Build history of the part. All positions in model axes, mm. A direction names the side the tool comes from. Give positions to 0.01 mm unless a question says otherwise; leave off trailing zeros. Write each loop counter-clockwise with the first axis right and the second up, starting at its lowest first coordinate (ties: lowest second). Pieces come first, ordered by that corner, then holes. Notation, with made-up numbers: (1.25, -1.5) -> (8.25, -1.5) arc R18 ccw to (8.25, 11.5) -> close; hole circle Ø4 at (81.5, 77). An arc over 180 degrees is marked (long way). Put each result on its own line as item: value. Start each with the question number.
Item 1: Slice it at A-A, the plane z = 28.5. List the corners of the cut face in (x, y).
Item 2: Two-plate mould, pull along X, no slides. Class faces 1 (the flat face through (-90.694, 2, 25)), 2 (the flat face through (-110, 2, 20.456)), 3 (the flat face through (-103, 3, 21.956)): pulls with the +X half, pulls with the -X half, needs draft (parallel to the pull), parting line crosses it, or undercut.
Item 3: Slice it at C-C, the plane z = 23.5. List the corners of the cut face in (x, y), plus the area to 3 significant figures.
Item 4: Slice it at B-B, the plane x = -95.25. List the corners of the cut face in (y, z).
Item 5: Flat gauge pins, fed straight in: pin 1 Ø4.5 at (x, z) = (-95.19, 24.96) entering from +Y; pin 2 Ø1.5 at (x, y) = (-103.5, 3) entering from -Z. Where does each tip first touch, or does it go through?
Item 6: Tool access for faces 4 (the flat face through (-99.694, 3, 21)), 5 (the flat face through (-95, 2, 29.456)), 6 (the flat face through (-99.694, 3, 29)): list every direction of +Z, -Z, +X, -X, +Y, -Y with a clear straight run to the whole face (end or side of a thin tool).
Item 7: Slice it at D-D, the plane y = 2.05. List the corners of the cut face in (x, z), plus the area to 3 significant figures.
Item 8: Drill centre lines: line 1 along X through (y, z) = (3.2, 26); line 2 along X through (y, z) = (1.55, 21.75); line 3 along X through (y, z) = (0.7, 24.75). Where is each one in solid material? Low to high.
```python
from build123d import *

# Parameters (mm, degrees)
SKETCH3_W           = 24
SKETCH3_H           = 9
BOSS_EXTRUDE2_DEPTH = 5
SKETCH4_R           = 1.7
SKETCH4_R_2         = 1
SKETCH4_W           = 6
SKETCH4_H           = 1.5
CUT_EXTRUDE1_DEPTH  = 5


with BuildPart() as part:
    # Sketch3 → Boss-Extrude2 (new body)
    with BuildSketch(Plane(origin=(0, 0, 0), x_dir=(1, 0, 0), z_dir=(0, 1, 0))):
        with Locations((-102.694405771, -24.955608755)):
            Rectangle(SKETCH3_W, SKETCH3_H)
    extrude(amount=BOSS_EXTRUDE2_DEPTH)

    # Sketch4 → Cut-Extrude1 (cut)
    with BuildSketch(Plane(origin=(0, 5, 0), x_dir=(1, 0, 0), z_dir=(0, 1, 0))):
        with Locations((-110.194405771, -24.955608755)):
            Circle(SKETCH4_R)
        with Locations((-95.194405771, -24.955608755)):
            Circle(SKETCH4_R)
        with Locations((-102.694405771, -24.955608755)):
            Circle(SKETCH4_R_2)
        with Locations((-102.694405771, -28.705608755)):
            Rectangle(SKETCH4_W, SKETCH4_H)
        with Locations((-102.694405771, -21.205608755)):
            Rectangle(SKETCH4_W, SKETCH4_H)
    extrude(amount=-CUT_EXTRUDE1_DEPTH, mode=Mode.SUBTRACT)


solid = part.part
```
Values follow:
1. outline: (-114.69, 0) -> (-105.69, 0) -> (-105.69, 5) -> (-114.69, 5) -> close; (-99.69, 0) -> (-90.69, 0) -> (-90.69, 5) -> (-99.69, 5) -> close
2. face 1: pulls with the +X half
2. face 2: needs draft
2. face 3: undercut
3. outline: (-114.69, 0) -> (-111.07, 0) -> (-111.07, 5) -> (-114.69, 5) -> close; (-109.32, 0) -> (-96.07, 0) -> (-96.07, 5) -> (-109.32, 5) -> close; (-94.32, 0) -> (-90.69, 0) -> (-90.69, 5) -> (-94.32, 5) -> close
3. area: 102 mm2
4. outline: (0, 20.46) -> (5, 20.46) -> (5, 23.26) -> (0, 23.26) -> close; (0, 26.65) -> (5, 26.65) -> (5, 29.46) -> (0, 29.46) -> close
5. pin 1: y = 5
5. pin 2: z = 21.96
6. face 4: -Z, +Y, -Y
6. face 5: +Z, +X, -X, +Y, -Y
6. face 6: +Z, +Y, -Y
7. outline: (-114.69, 20.46) -> (-105.69, 20.46) -> (-105.69, 21.96) -> (-99.69, 21.96) -> (-99.69, 20.46) -> (-90.69, 20.46) -> (-90.69, 29.46) -> (-99.69, 29.46) -> (-99.69, 27.96) -> (-105.69, 27.96) -> (-105.69, 29.46) -> (-114.69, 29.46) -> close; hole circle Ø3.4 at (-110.19, 24.96); hole circle Ø2 at (-102.69, 24.96); hole circle Ø3.4 at (-95.19, 24.96)
7. area: 177 mm2
8. line 1: -114.69 to -111.54, -108.85 to -96.54, -93.85 to -90.69
8. line 2: -114.69 to -105.69, -99.69 to -90.69
8. line 3: -114.69 to -111.88, -108.51 to -103.67, -101.72 to -96.88, -93.51 to -90.69
